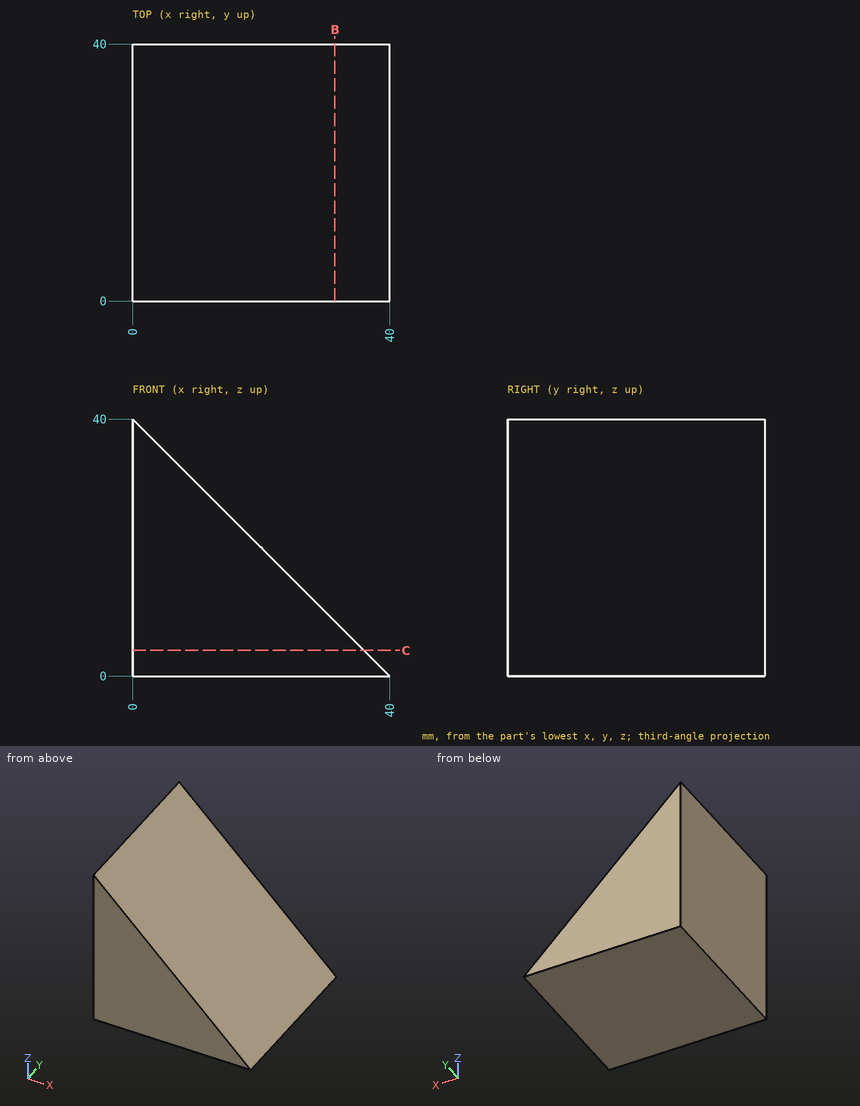
Input: dimensioned drawing with shaded views. Units: mm. Origin: part minimum x, y, z. Coordinates: 2 decimals unless noted, no trailing zeros. Write each loop counter-clockwise with the first axis right and the second up, starting at its lowest first coordinate (ties: lowest second). Pieces come first, ordered by that corner, then holes. Notation, with made-up numbers: M -5.5,21.25 L 41.5,21.25 A7 ccw 41.5,25.25 Z; hole C 41,49 d6. An arc over 180 degrees is marked long. Answer as a JSON object with one key per item and string values. Group by question number.
(1) Ray query, line 1 along X through (y, z) = (36.5, 19); line 2 along X through (y, z) = (10.5, 6); line 3 along Z through (x, y) = (22.5, 33). Return the intervals inside material, ascending. Write a range as [from, to].
(2) Contact query for flat-ended pins moving along their axis: P1, Ø1, axis at y = 9.5, z = 33.5, coming from the +X side; P2, Ø1, axis at y = 31.5, z = 30.5, coming from the +X side; P3, Ø3, axis at y = 12.5, z = 29, coming from the +X side. Output: stop coordinate, or through.
(3) Section C-C on z = 4. Output: boundary loops of the cut face in (x, y).
(4) Section B-B on x = 31.5. Output: boundary loops of the cut face in (y, z), plus the area to 3 significant figures.
Result set:
{
 "1": {"line 1": "x = [0, 21]", "line 2": "x = [0, 34]", "line 3": "z = [0, 17.5]"},
 "2": {"P1": "stops at x = 7", "P2": "stops at x = 10", "P3": "stops at x = 12.5"},
 "3": {"outline": "M 0,0 L 36,0 L 36,40 L 0,40 Z"},
 "4": {"outline": "M 0,0 L 40,0 L 40,8.5 L 0,8.5 Z", "area": "340 mm2"}
}
